from build123d import *

# Parameters (mm, degrees)
SKETCH_1_R               = 26.45
SKETCH_1_R_2             = 17.6
EXTRUDE_1_DEPTH          = 1.6
SKETCH_2_W               = 4.9
SKETCH_2_H               = 4.9
EXTRUDE_2_DEPTH          = 1.5
PATTERN_CIRCULAR_1_COUNT = 12


with BuildPart() as part:
    # 草图1 → 凸台-拉伸1 (new body)
    with BuildSketch(Plane(origin=(0, 0, 0), x_dir=(1, 0, 0), z_dir=(0, 1, 0))):
        Circle(SKETCH_1_R)
        Circle(SKETCH_1_R_2, mode=Mode.SUBTRACT)
    extrude(amount=EXTRUDE_1_DEPTH)

    # 草图2 → 凸台-拉伸2 (add)
    with BuildSketch(Plane(origin=(0, 1.6, 0), x_dir=(1, 0, 0), z_dir=(0, 1, 0))):
        with Locations((-22.65, 0)):
            Rectangle(SKETCH_2_W, SKETCH_2_H)
    extrude_2 = extrude(amount=EXTRUDE_2_DEPTH)

    # 阵列(圆周)1: 凸台-拉伸2 ×12 about axis
    pattern_circular_1_axis = Axis((0, 0, 0), (0, 1, 0))
    for i in range(1, PATTERN_CIRCULAR_1_COUNT):
        add(extrude_2.rotate(pattern_circular_1_axis, i * 360 / PATTERN_CIRCULAR_1_COUNT))


solid = part.part
Build history of the part. All positions in model axes, mm. A direction names the side the tool comes from. Round coordinates to 2 decimals unless told otherwise and drop trailing zeros. Write each loop counter-clockwise with the first axis right and the second up, starting at its lowest first coordinate (ties: lowest second). Pieces come first, ordered by that corner, then holes. Notation, with made-up numbers: M -31.5,7 L -1.5,7 A20 cw -1.5,36 Z; hole C 0.25,32.5 d3. An arc over 180 degrees is marked long. Answer in a Markdown table with one row per item.
1. Saw through at D-D (x = -5.5). List the corners of the cut face in (y, z).
Geometry check:
| item | result |
|---|---|
| outline | M 0,-25.87 L 1.6,-25.87 L 1.6,-16.72 L 0,-16.72 Z; M 0,16.72 L 1.6,16.72 L 1.6,25.87 L 0,25.87 Z |
2. Which spindle directions (+Z, -Z, +X, -X, +Y, -Y) get a long thin tool onto all of the face, cutting with end or side? Do faces 4 (the face through (-23, 2, -2.45)), 5 (the face through (13.464, 2.34, -18.42)), 6 (the face through (25.1, 2, 0)), 7 (the face through (0, 2, -20.2)), 8 (the face through (-18.42, 2.34, -13.464)). Say none if no direction does.
Geometry check:
| item | result |
|---|---|
| face 4 | +X, -X, +Y |
| face 5 | +X, +Y |
| face 6 | +Z, -Z, +X, +Y |
| face 7 | +Y |
| face 8 | -Z, +Y |
3. Mould opens along X. For faces 1 (the face through (20, 3.1, -11)), 2 (the face through (-25.1, 2, 0)), 3 (the face through (18.42, 2.34, -13.464)) say: +X half, -X half, draft (parallel to the pull), parting line (faces both ways), or undercut.
Geometry check:
| item | result |
|---|---|
| face 1 | draft |
| face 2 | -X half |
| face 3 | undercut |
4. Probe L1, parallel to X at y = 0.75, z = 0; L2, parallel to Z at x = 1.5, y = 1.85; L3, parallel to Z at x = 22, y = 2.1. List the from-to ranges inside material, lowest first. Write a range as [from, to].
Geometry check:
| item | result |
|---|---|
| L1 | [-26.45, -17.6], [17.6, 26.45] |
| L2 | [-25.1, -20.2], [20.2, 25.1] |
| L3 | [-12.09, -9.87], [-2.45, 2.45], [9.87, 12.09] |
5. Flat gauge pins, fed straight in: P1, Ø1.2, axis at x = 23.5, y = 2, coming from the +Z side; P2, Ø1, axis at y = 1, z = -13, coming from the -X side; P3, Ø1.2, axis at y = 2, z = 22.5, coming from the -X side; P4, Ø8, axis at x = 6.5, z = 19.5, coming from the +Y side. Where does each tip first touch, or does it go through?
Geometry check:
| item | result |
|---|---|
| P1 | z = 12.97 |
| P2 | x = -23.31 |
| P3 | x = -14.6 |
| P4 | y = 3.1 |
6. Saw through at A-A (x = 0). List the corners of the cut face in (y, z), and give its area (3 significant figures).
Geometry check:
| item | result |
|---|---|
| outline | M 0,-26.45 L 1.6,-26.45 L 1.6,-25.1 L 3.1,-25.1 L 3.1,-20.2 L 1.6,-20.2 L 1.6,-17.6 L 0,-17.6 Z; M 0,17.6 L 1.6,17.6 L 1.6,20.2 L 3.1,20.2 L 3.1,25.1 L 1.6,25.1 L 1.6,26.45 L 0,26.45 Z |
| area | 43.0 mm2 |
7. Saw through at C-C (y = 0.75). List the corners of the cut face in (x, z).
Geometry check:
| item | result |
|---|---|
| outline | C 0,0 d52.9; hole C 0,0 d35.2 |
8. Saw through at B-B (z = 0). List the corners of the cut face in (x, y).
Geometry check:
| item | result |
|---|---|
| outline | M -26.45,0 L -17.6,0 L -17.6,1.6 L -20.2,1.6 L -20.2,3.1 L -25.1,3.1 L -25.1,1.6 L -26.45,1.6 Z; M 17.6,0 L 26.45,0 L 26.45,1.6 L 25.1,1.6 L 25.1,3.1 L 20.2,3.1 L 20.2,1.6 L 17.6,1.6 Z |
